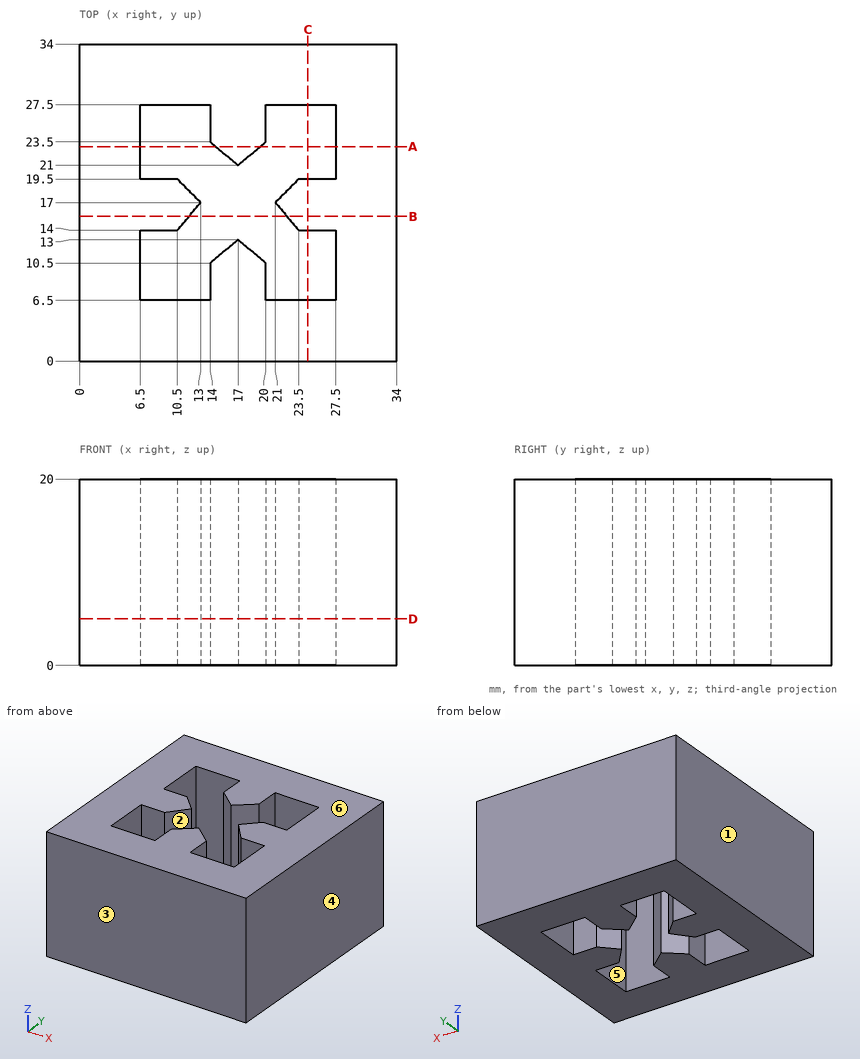
Design review of the part shown in the three views and the two pictorial views. Dimensions are in mm from the part's minimum x, y and z. A direction names the side the tool comes from. Round coordinates to 2 decimals unless told otherwise and drop trailing zeros. Loops run counter-clockwise (first coordinate to the right, second up) from the corner with the lowest first, then second, coordinate; pieces in that order, holes last. Notation, with made-up numbers: M 50,82.5 L 82,82.5 A29 ccw 82,102.5 Z; hole C 45.5,60.5 d11. An arc over 180 degrees is marked long. Answer as a JSON object with one key per item and string values.
Item 1: We need section D-D on z = 5. Give the boundary of the cut face in (x, y), and give its area (3 significant figures).
Answer sheet:
{"outline": "M 0,0 L 34,0 L 34,34 L 0,34 Z; hole M 6.5,6.5 L 14,6.5 L 14,10.5 L 17,13 L 20,10.5 L 20,6.5 L 27.5,6.5 L 27.5,14 L 23.5,14 L 21,17 L 23.5,19.5 L 27.5,19.5 L 27.5,27.5 L 20,27.5 L 20,23.5 L 17,21 L 14,23.5 L 14,27.5 L 6.5,27.5 L 6.5,19.5 L 10.5,19.5 L 13,17 L 10.5,14 L 6.5,14 Z", "area": "836 mm^2"}
Item 2: We need section A-A on y = 23. Give the boundary of the cut face in (x, z), and give its area (3 significant figures).
Answer sheet:
{"outline": "M 0,0 L 6.5,0 L 6.5,20 L 0,20 Z; M 14.6,0 L 19.4,0 L 19.4,20 L 14.6,20 Z; M 27.5,0 L 34,0 L 34,20 L 27.5,20 Z", "area": "356 mm^2"}
Item 3: Wall thickness on L1, parallel to X at y = 8.5, z = 6.25; L2, parallel to Y at x = 27, z = 18; L3, parallel to Y at x = 20.5, z = 2.5: over which ranges is each line inside the solid? List them lowest first. Write a range as from..to.
Answer sheet:
{"L1": "x = 0..6.5, 14..20, 27.5..34", "L2": "y = 0..6.5, 14..19.5, 27.5..34", "L3": "y = 0..6.5, 27.5..34"}
Item 4: The part is to be moulded in two halves that separate along X. For the marked faces 1, 2, 3 and 4, say which applies: pulls with the +X half, pulls with the -X half, needs draft (parallel to the pull), parting line crosses it, or undercut.
Answer sheet:
{"face 1": "pulls with the -X half", "face 2": "undercut", "face 3": "needs draft", "face 4": "pulls with the +X half"}
Item 5: We need section B-B on y = 15.5. Give the boundary of the cut face in (x, z).
Answer sheet:
{"outline": "M 0,0 L 11.75,0 L 11.75,20 L 0,20 Z; M 22.25,0 L 34,0 L 34,20 L 22.25,20 Z"}
Item 6: Machinability: for the marked faces 5 and 6, which of the approach directions +Z, -Z, +X, -X, +Y, -Y give a long, thin tool a straight path to every point of the face, cutting with its end or side? Answer none if there is none.
Answer sheet:
{"face 5": "+Z, -Z", "face 6": "+Z, +X, -X, +Y, -Y"}
Item 7: We need section C-C on x = 24.5. Give the boundary of the cut face in (y, z).
Answer sheet:
{"outline": "M 0,0 L 6.5,0 L 6.5,20 L 0,20 Z; M 14,0 L 19.5,0 L 19.5,20 L 14,20 Z; M 27.5,0 L 34,0 L 34,20 L 27.5,20 Z"}
Item 8: Clearance check with a flat-ended pin moving along its axis: P1, Ø1.5, axis at x = 11.5, y = 23.5, coming from the +Z side. State where the tip first meets the part, or that it passes through.
Answer sheet:
{"P1": "passes through"}
